Autodesk Inventor part; units mm, degrees
sketch "Sketch1" plane through (0, 0, 0) normal (0, 0, 1) x (1, 0, 0)
  line L0 (-5.2, 0) -> (-5.2, 5.2)
  line L1 (0, 14.64) -> (0, -2.44)
  line L2 (-5.2, 0) -> (-6.2, 0)
  line L3 (-6.2, 0) -> (-7.2, 1)
  line L4 (-8.64, 0) -> (1.44, 0)
  line L5 (-7.2, 1) -> (-7.2, 6.2)
  line L6 (-5.2, 5.2) -> (-3.2, 5.2)
  line L7 (-3.2, 5.2) -> (-3.2, 7.6)
  line L8 (-3.2, 7.6) -> (-1.4, 7.6)
  line L9 (0, 7.2) -> (0, 12.2)
  line L10 (-1.4, 10) -> (-2.4, 10)
  line L11 (-2.4, 10) -> (-7.2, 6.2)
  line L12 (0, -2.44) -> (0, 14.64)
  line L13 (-1.4, 7.6) -> (-1.4, 10)
  point P0 (0, 0)
  dimension "d0" = 5.2
  dimension "d1" = 5.2
  dimension "d2" = 1
  dimension "d3" = 1
  dimension "d5" = 5.2
  dimension "d6" = 3.2
  dimension "d7" = 2.4
  dimension "d8" = 0
  dimension "d11" = 2.4
  dimension "d21" = 1.4
  dimension "d22" = 2
  dimension "d23" = 2.4
revolve "Revolution1" add sketch "Sketch1" angle 360 about axis through (0, -10, 0) along (0, 1, 0)
properties part number "magnet-holder" material "PET Plastic"
Input: part model. Units: mm. Frame: model coordinates. A direction names the side the tool comes from. Give positions to 0.01 mm unless a question says otherwise; leave off trailing zeros. Loops run counter-clockwise (first coordinate to the right, second up) from the corner with the lowest first, then second, coordinate; pieces in that order, holes last. Notation, with made-up numbers: (25, -32.75) -> (42, -32.75) arc R6 ccw to (42, -26.75) -> close; hole circle Ø11 at (-14.75, -39). An arc over 180 degrees is marked (long way). Answer as a JSON object with one key per item and string values. Group by question number.
Item 1: Cut plane D-D, the plane y = 7. Return the cut outline in (x, z), and give its area (3 significant figures).
Item 2: Cut plane B-B, the plane z = 0. Return the cut outline in (x, y).
Item 3: Pin query (flat end, axial travel): P1, Ø1.5, axis at y = 3.5, z = -1, coming from the +X side; P2, Ø5, axis at x = 0.5, z = -1, coming from the -Y side; P3, Ø4, axis at x = -5, y = 5.5, coming from the +Z side. Return the tip coordinate at first contact, or that it passes through.
Item 4: Line query: probe 1 along Z at (x, y) = (0, 3.2); probe 2 along Z at (x, y) = (0.5, 7.75); probe 3 along Y at (x, z) = (-1.75, 0). Output: solid intervals per line, ascending.
Item 5: Cut plane C-C, the plane y = 3.5. Return the cut outline in (x, z).
Item 6: Cut plane A-A, the plane x = 0. Return the cut outline in (y, z).
Item 7: Pull-direction query (X, two-part tool) for faces 3 (the flat face through (0, 10, -2)), 4 (the cylindrical face through (-6.87, 3.64, 2.16)), 5 (the flat face through (-1.4, 7.6, -0.7)), 6 (the flat face through (-3.4, 5.2, 0.1)); classes: released by +X, released by -X, zero draft, split by the parting line, or undercut.
Item 8: Reachability of faces 1 (the cylindrical face through (1.4, 8.82, 0.06)), 2 (the cylindrical face through (0.677, 2.636, 5.156)) from +Z, -Z, +X, -X, +Y, -Y: full face, straight path, thin tool, end or side. Return the list, or none.
Checks:
{
 "1": {"outline": "circle Ø12.38 at (0, 0); hole circle Ø6.4 at (0, 0)", "area": "88.2 mm²"},
 "2": {"outline": "(-7.2, 1) -> (-6.2, 0) -> (-5.2, 0) -> (-5.2, 5.2) -> (-3.2, 5.2) -> (-3.2, 7.6) -> (-1.4, 7.6) -> (-1.4, 10) -> (-2.4, 10) -> (-7.2, 6.2) -> close; (1.4, 7.6) -> (3.2, 7.6) -> (3.2, 5.2) -> (5.2, 5.2) -> (5.2, 0) -> (6.2, 0) -> (7.2, 1) -> (7.2, 6.2) -> (2.4, 10) -> (1.4, 10) -> close"},
 "3": {"P1": "stops at x = 7.2", "P2": "stops at y = 5.2", "P3": "stops at z = 6.55"},
 "4": {"probe 1": "z = -7.2 to -5.2, 5.2 to 7.2", "probe 2": "z = -5.22 to -1.31, 1.31 to 5.22", "probe 3": "y = 7.6 to 10"},
 "5": {"outline": "circle Ø14.4 at (0, 0); hole circle Ø10.4 at (0, 0)"},
 "6": {"outline": "(0, -6.2) -> (1, -7.2) -> (6.2, -7.2) -> (10, -2.4) -> (10, -1.4) -> (7.6, -1.4) -> (7.6, -3.2) -> (5.2, -3.2) -> (5.2, -5.2) -> (0, -5.2) -> close; (0, 5.2) -> (5.2, 5.2) -> (5.2, 3.2) -> (7.6, 3.2) -> (7.6, 1.4) -> (10, 1.4) -> (10, 2.4) -> (6.2, 7.2) -> (1, 7.2) -> (0, 6.2) -> close"},
 "7": {"face 3": "zero draft", "face 4": "split by the parting line", "face 5": "undercut", "face 6": "undercut"},
 "8": {"face 1": "+Y, -Y", "face 2": "-Y"}
}
